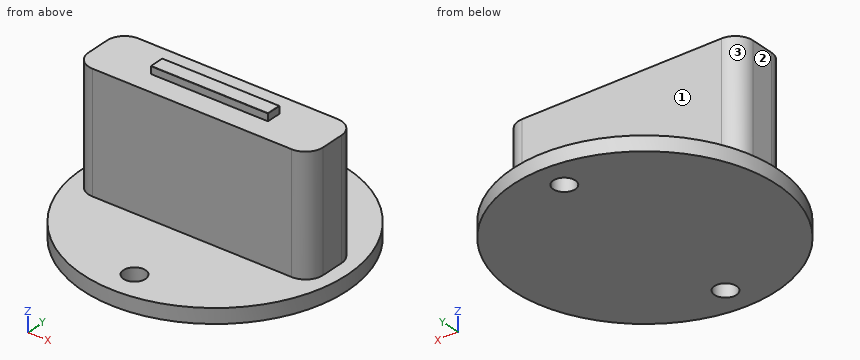
from build123d import *

# Parameters (mm, degrees)
F0_W     = 101.6
F0_H     = 25.4
F1_DEPTH = 50.8
F2_W     = 50.8
F2_H     = 6.35
F3_DEPTH = 3.175
F4_R     = 57.15
F5_DEPTH = 6.35
F6_R     = 4.7625
F7_DEPTH = 25.4
F8_R     = 7.62
F9_R     = 0.127


with BuildPart() as f1:
    # F0 (on Top) → F1 (new body)
    with BuildSketch(Plane.XY):
        Rectangle(F0_W, F0_H)
    extrude(amount=F1_DEPTH)

    # F2 (on face) → F3 (join)
    with BuildSketch(Plane.XY.offset(50.8)):
        Rectangle(F2_W, F2_H)
    extrude(amount=F3_DEPTH)

    # F4 (on face) → F5 (join)
    with BuildSketch(Plane(origin=(0, 0, 0), x_dir=(1, 0, 0), z_dir=(0, 0, -1))):
        Circle(F4_R)
    extrude(amount=F5_DEPTH)

    # F6 (on face) → F7 (cut)
    with BuildSketch(Plane(origin=(0, 0, -6.35), x_dir=(1, 0, 0), z_dir=(0, 0, -1))):
        with Locations((0, 44.45)):
            Circle(F6_R)
        with Locations((0, -44.45)):
            Circle(F6_R)
    extrude(amount=-F7_DEPTH, mode=Mode.SUBTRACT)

    # F8
    f8_edges = [f1.edges().sort_by_distance(p)[0] for p in [
        (50.8, -12.7, 25.4),
        (50.8, 12.7, 25.4),
        (-50.8, -12.7, 25.4),
        (-50.8, 12.7, 25.4),
    ]]
    fillet(f8_edges, radius=F8_R)

    # F9
    f9_edges = [f1.edges().sort_by_distance(p)[0] for p in [
        (0, 3.175, 53.975),
        (-25.4, 0, 53.975),
        (0, -3.175, 53.975),
        (25.4, 0, 53.975),
        (25.4, -3.175, 52.3875),
        (25.4, 3.175, 52.3875),
        (-25.4, -3.175, 52.3875),
        (-25.4, 3.175, 52.3875),
    ]]
    fillet(f9_edges, radius=F9_R)


solid = f1.part
Design review of the part built by this model. Coordinates are the model's own, in mm. Face numbers are marked on the shaded views. A direction names the side the tool comes from. Give positions to 0.01 mm unless a question says otherwise; leave off trailing zeros. Order: outer loops, then holes, each group sorted by start corner. A loop starts at its lowest first (then second) coordinate and runs counter-clockwise, first axis right, second up. Notation, with made-up numbers: (-13, 17) - (-1, 17) arc R30 ccw to (-1, 53) - close; hole circle Ø10 at (10, 80.5). An arc over 180 degrees is marked (long way). Write item = value, one per line. Start each with the question number.
Q1. Tool access review of the marked faces 1, 2 and 3: name each direction out of +Z, -Z, +X, -X, +Y, -Y from which nothing blocks a thin tool from reaching the whole face with its end or side.
Q2. To check wall thickness, follow L1, parallel to Y at x = 0, z = -4; L2, parallel to Z at x = 5.5, y = -41.5; L3, parallel to X at y = -44, z = -4. State the ranges of each line that lie inside material, in increasing order. Write a range as from..to.
Q3. We need section C-C on y = 0. State the section outline as (x, z) points (3 decimals).
Q4. Clearance check with flat-ended pins moving along their axes: pin 1 Ø6 at (x, z) = (18, 17.5) entering from -Y; pin 2 Ø0.9 at (y, z) = (0.5, 53) entering from +X; pin 3 Ø0.9 at (x, z) = (-10.5, 52) entering from -Y (3 decimals); pin 4 Ø5.5 at (x, y) = (0, -44.45) entering from -Z. State where each tip first meets the part, or that it passes through.
Q5. We need section D-D on x = -49. State the section outline as (y, z) points.
Q6. We need section B-B on z = 16.5. State the section outline as (x, y) points.
Q7. We need section A-A on y = 44.45. State the section outline as (x, z) points, plus the area to 3 significant figures.
Working result:
q1.face_1 = +Z, +X, -X, +Y
q1.face_2 = +Z, -X, +Y, -Y
q1.face_3 = +Z, -X, +Y
q2.L1 = -57.15..-49.21, -39.69..39.69, 49.21..57.15
q2.L2 = -6.35..0
q2.L3 = -36.47..-4.74, 4.74..36.47
q3.outline = (-57.15, -6.35) - (57.15, -6.35) - (57.15, 0) - (50.8, 0) - (50.8, 50.8) - (25.4, 50.8) - (25.4, 53.848) arc R0.127 ccw to (25.273, 53.975) - (-25.273, 53.975) arc R0.127 ccw to (-25.4, 53.848) - (-25.4, 50.8) - (-50.8, 50.8) - (-50.8, 0) - (-57.15, 0) - close
q4.pin_1 = -12.7
q4.pin_2 = 25.4
q4.pin_3 = -3.175
q4.pin_4 = through
q5.outline = (-29.41, -6.35) - (29.41, -6.35) - (29.41, 0) - (10, 0) - (10, 50.8) - (-10, 50.8) - (-10, 0) - (-29.41, 0) - close
q6.outline = (-50.8, -5.08) arc R7.62 ccw to (-43.18, -12.7) - (43.18, -12.7) arc R7.62 ccw to (50.8, -5.08) - (50.8, 5.08) arc R7.62 ccw to (43.18, 12.7) - (-43.18, 12.7) arc R7.62 ccw to (-50.8, 5.08) - close
q7.outline = (-35.92, -6.35) - (-4.76, -6.35) - (-4.76, 0) - (-35.92, 0) - close; (4.76, -6.35) - (35.92, -6.35) - (35.92, 0) - (4.76, 0) - close
q7.area = 396 mm²
